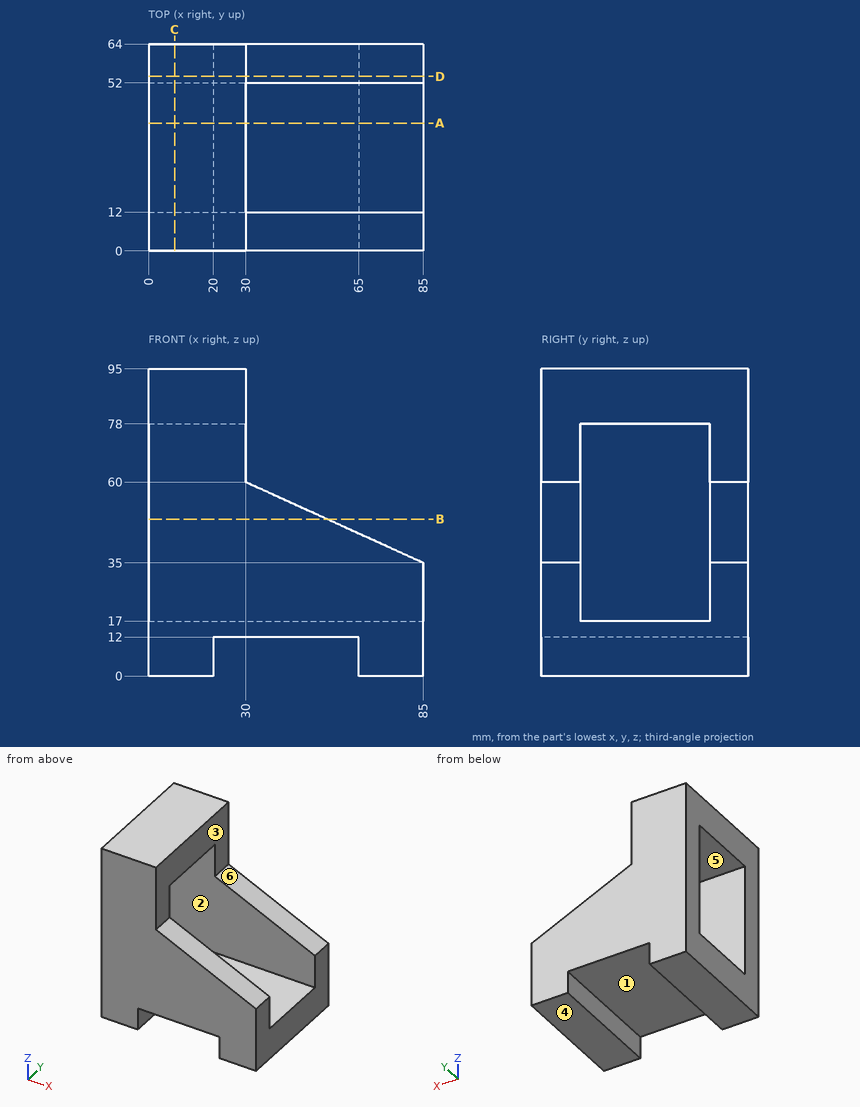
Could you check a few things on this drawing? It's one solid part, dimensions in mm from its lowest x, y, z. A direction names the side the tool comes from. Round coordinates to 2 decimals unless told otherwise and drop trailing zeros. Order: outer loops, then holes, each group sorted by start corner. A loop starts at its lowest first (then second) coordinate and runs counter-clockwise, first axis right, second up.
Q1. Which directions (+Z, -Z, +X, -X, +Y, -Y) give clear straight access to the entire face, cutting with the end or side of a thin tool? Please do the marked faces 1, 2 and 3.
Geometry says:
face 1: -Z, +Y, -Y
face 2: +X, -X
face 3: +Z, +X, +Y, -Y
Q2. Imagine slicing it at B-B, the plane z = 48.5. List the corners of the cut face in (x, y) for me.
Geometry says:
outline: (0, 0) - (55.3, 0) - (55.3, 12) - (0, 12) - close; (0, 52) - (55.3, 52) - (55.3, 64) - (0, 64) - close
Q3. Imagine slicing it at A-A, the plane y = 39.5. List the corners of the cut face in (x, z) for me, then the cut area to 4 significant figures.
Geometry says:
outline: (0, 0) - (20, 0) - (20, 12) - (65, 12) - (65, 0) - (85, 0) - (85, 17) - (0, 17) - close; (0, 78) - (30, 78) - (30, 95) - (0, 95) - close
area: 1,415 mm2
Q4. Thinking about a two-plate mould opening in Z: for the marked faces 4, 5 and 6, which applies, released by +Z, released by -Z, zero draft, split by the parting line, or undercut?
Geometry says:
face 4: released by -Z
face 5: undercut
face 6: released by +Z
Q5. I'm going to push flat-ended pins straight in: P1, Ø17.5, axis at y = 33, z = 74, coming from the +X side; P2, Ø8, axis at x = 41, y = 57.5, coming from the -Z side. Where does each tip first touch, or does it pass through?
Geometry says:
P1: stops at x = 30
P2: stops at z = 12
Q6. Imagine slicing it at D-D, the plane y = 54. List the corners of the cut face in (x, z) for me.
Geometry says:
outline: (0, 0) - (20, 0) - (20, 12) - (65, 12) - (65, 0) - (85, 0) - (85, 35) - (30, 60) - (30, 95) - (0, 95) - close
Q7. Imagine slicing it at C-C, the plane x = 8. List the corners of the cut face in (y, z) for me, then the cut area to 3 significant figures.
Geometry says:
outline: (0, 0) - (64, 0) - (64, 95) - (0, 95) - close; hole (12, 17) - (52, 17) - (52, 78) - (12, 78) - close
area: 3,640 mm2
Q8. Please list where these lines run through material, in increasing order: probe 1 along Y at (x, z) = (27.5, 55.5); probe 2 along Z at (x, y) = (26, 17); probe 3 along Z at (x, y) = (32, 43.5).
Geometry says:
probe 1: y = 0 to 12, 52 to 64
probe 2: z = 12 to 17, 78 to 95
probe 3: z = 12 to 17
